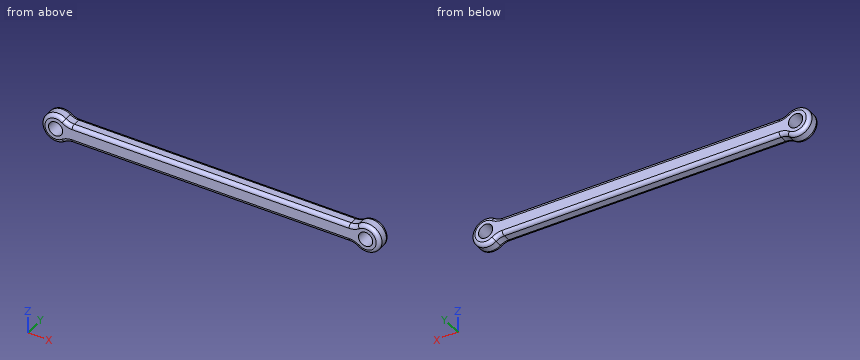
from build123d import *

# Parameters (mm, degrees)
SKETCH1_R           = 5
BOSS_EXTRUDE1_DEPTH = 10
FILLET1_R           = 2.54
SCALE1_SCALE        = 0.66


with BuildPart() as part:
    # Sketch1 → Boss-Extrude1 (new body)
    with BuildSketch(Plane(origin=(0, 0, 0), x_dir=(1, 0, 0), z_dir=(0, 1, 0))):
        with BuildLine():
            Line((-42.950776184, -6.25), (152.170776184, -6.25))
            ThreePointArc((152.170776184, -6.25), (155.232638362, -6.730283618), (158.000388092, -8.125))
            ThreePointArc((158.000388092, -8.125), (173.83, 0), (158.000388092, 8.125))
            ThreePointArc((158.000388092, 8.125), (155.232638362, 6.730283618), (152.170776184, 6.25))
            Line((152.170776184, 6.25), (-42.950776184, 6.25))
            ThreePointArc((-42.950776184, 6.25), (-46.012638362, 6.730283618), (-48.780388092, 8.125))
            ThreePointArc((-48.780388092, 8.125), (-64.61, 0), (-48.780388092, -8.125))
            ThreePointArc((-48.780388092, -8.125), (-46.012638362, -6.730283618), (-42.950776184, -6.25))
        make_face()
        with Locations((-54.61, 0)):
            Circle(SKETCH1_R, mode=Mode.SUBTRACT)
        with Locations((163.83, 0)):
            Circle(SKETCH1_R, mode=Mode.SUBTRACT)
    extrude(amount=BOSS_EXTRUDE1_DEPTH)

    # Fillet1
    fillet1_edges = [part.edges().sort_by_distance(p)[0] for p in [
        (-46.012638362, 10, 6.730283618),
        (-64.61, 0, 0),
        (-46.012638362, 0, -6.730283618),
        (54.61, 10, 6.25),
        (155.232638362, 10, 6.730283618),
        (173.83, 10, 0),
        (155.232638362, 10, -6.730283618),
        (54.61, 10, -6.25),
        (-46.012638362, 10, -6.730283618),
        (-64.61, 10, 0),
        (54.61, 0, -6.25),
        (155.232638362, 0, -6.730283618),
        (173.83, 0, 0),
        (155.232638362, 0, 6.730283618),
        (54.61, 0, 6.25),
        (-46.012638362, 0, 6.730283618),
    ]]
    fillet(fillet1_edges, radius=FILLET1_R)


with BuildPart() as part_1:
    # Scale1: scaled about (54.61, 5, 0)
    add(part.part.scale(SCALE1_SCALE).moved(Location((18.5674, 1.7, 0))))


solid = part_1.part
Work out the finished part from the listing and answer in its coordinate system (mm). Round coordinates to 2 decimals unless told otherwise and drop trailing zeros. Write each loop counter-clockwise with the first axis right and the second up, starting at its lowest first coordinate (ties: lowest second). Pieces come first, ordered by that corner, then holes. Notation, with made-up numbers: (11.25, -10.75) -> (35.25, -10.75) arc R24 cw to (35.25, 9.25) -> close; hole circle Ø11 at (61.25, -16.5). An arc over 180 degrees is marked (long way). Write each question's results on one line, items separated by ' | '.
Item 1: Find the intervals of material crossed by line 1 along X through (y, z) = (4, 0); line 2 along X through (y, z) = (4.5, -2); line 3 along Z through (x, y) = (87, 4.75) (3 decimals), in increasing order. Write a range as [from, to].
Result set:
line 1: [-24.08, -20.78], [-14.18, 123.4], [130, 133.3] | line 2: [-23.76, -20.1], [-14.85, 124.07], [129.32, 132.98] | line 3: [-4.125, 4.125]
Item 2: A cutting plane is placed at A-A, the plane z = 0. Determine the outline of the cut face in (x, y), plus the area to 3 significant figures.
Result set:
outline: (-24.08, 3.38) arc R1.68 ccw to (-22.4, 1.7) -> (-20.78, 1.7) -> (-20.78, 8.3) -> (-22.4, 8.3) arc R1.68 ccw to (-24.08, 6.62) -> close; (-14.18, 1.7) -> (123.4, 1.7) -> (123.4, 8.3) -> (-14.18, 8.3) -> close; (130, 1.7) -> (131.62, 1.7) arc R1.68 ccw to (133.3, 3.38) -> (133.3, 6.62) arc R1.68 ccw to (131.62, 8.3) -> (130, 8.3) -> close | area: 949 mm^2
Item 3: A cutting plane is placed at C-C, the plane x = 17. Determine the outline of the cut face in (y, z) (3 decimals).
Result set:
outline: (1.7, -2.449) arc R1.676 ccw to (3.376, -4.125) -> (6.624, -4.125) arc R1.676 ccw to (8.3, -2.449) -> (8.3, 2.449) arc R1.676 ccw to (6.624, 4.125) -> (3.376, 4.125) arc R1.676 ccw to (1.7, 2.449) -> close
Item 4: A cutting plane is placed at B-B, the plane y = 5.25. Determine the outline of the cut face in (x, z) (1 decimal).
Result set:
outline: (-13.6, -5.4) arc R6.6 cw to (-9.8, -4.1) -> (119, -4.1) arc R6.6 cw to (122.8, -5.4) arc R6.6 ccw (long way) to (122.8, 5.4) arc R6.6 cw to (119, 4.1) -> (-9.8, 4.1) arc R6.6 cw to (-13.6, 5.4) arc R6.6 ccw (long way) to start; hole circle Ø6.6 at (-17.5, 0); hole circle Ø6.6 at (126.7, 0)
Item 5: Flat-ended cylindrical pins translate along their axes: P1, Ø7.5, axis at x = -17.48, z = 0, coming from the +Y side; P2, Ø3.5, axis at x = 77.5, y = 5.5, coming from the +Z side (3 decimals); P3, Ø1, axis at x = 66, y = 5.5, coming from the -Z side (3 decimals). Find the tip coordinate at first contact, or state that the pin passes through.
Result set:
P1: y = 8.3 | P2: z = 4.125 | P3: z = -4.125
